Autodesk Inventor part; units mm, degrees
ref_plane "YZ Plane" through (0, 0, 0) normal (1, 0, 0) x (0, 1, 0)
ref_plane "XZ Plane" through (0, 0, 0) normal (0, 1, 0) x (-1, 0, 0)
ref_plane "XY Plane" through (0, 0, 0) normal (0, 0, 1) x (1, 0, 0)
sketch "Sketch1" plane through (0, 0, 0) normal (0, 0, 1) x (1, 0, 0)
  circle A0 centre (0, 0) radius 37.5
  dimension "d0" = 75
extrude "Extrusion1" add sketch "Sketch1" along normal blind 1
sketch "Sketch2" plane through (0, 0, 1) normal (0, 0, 1) x (1, 0, 0)
  line L0 (-10, -10) -> (10, -10)
  line L1 (10, -10) -> (10, 10)
  line L2 (10, 10) -> (-10, 10)
  line L3 (-10, 10) -> (-10, -10)
  line L4 (-10, 10) -> (10, 10)
  line L5 (10, 10) -> (10, 36.1421)
  line L6 (-10, 36.1421) -> (-10, 10)
  line L7 (10, 10) -> (36.1421, 10)
  line L8 (36.1421, -10) -> (10, -10)
  line L9 (10, -10) -> (10, 10)
  line L10 (-10, -10) -> (10, -10)
  line L11 (10, -10) -> (10, -36.1421)
  line L12 (-10, -36.1421) -> (-10, -10)
  line L13 (-10, -10) -> (-36.1421, -10)
  line L14 (-36.1421, 10) -> (-10, 10)
  line L15 (-10, 10) -> (-10, -10)
  line L16 (35.8504, 11) -> (10, 11)
  line L17 (9, 9) -> (9, -9)
  line L18 (10, -11) -> (35.8504, -11)
  line L19 (11, 10) -> (11, 35.8504)
  line L20 (-11, 35.8504) -> (-11, 10)
  line L21 (-10, 11) -> (-35.8504, 11)
  line L22 (-35.8504, -11) -> (-10, -11)
  line L23 (-9, -9) -> (-9, 9)
  line L24 (-9, -9) -> (9, -9)
  line L25 (11, -10) -> (11, -35.8504)
  line L26 (-11, -35.8504) -> (-11, -10)
  line L27 (-9, 9) -> (9, 9)
  line L28 (9, 9) -> (9, -9)
  line L29 (9, -9) -> (-9, -9)
  line L30 (10, -10) -> (9, -9) construction
  line L31 (-9, 9) -> (-10, 10) construction
  line L32 (-10, -10) -> (-9, -9) construction
  line L33 (9, 9) -> (10, 10) construction
  circle A0 centre (0, 0) radius 37.5
  line L34 (-9, -49.0456) -> (-11, -49.0456)
  point P0 (-11, -11)
  point P1 (11, -11)
  point P2 (-11, 11)
  point P3 (11, 11)
  dimension "d3" = 20
  dimension "d4" = 20
  dimension "d5" = 1
  dimension "d6" = 1
  dimension "d7" = 1
  dimension "d8" = 1
  dimension "d9" = 1
extrude "Extrusion2" add sketch "Sketch2" along normal blind 23 contours L3 L2 L1 L0 | L12 L22 L26 L13 | L8 L25 L18 L11 | L14 L20 L21 L6 | L12 A0 L26 L22 | L26 L22 A0 L13 | L5 L16 L19 L7 | L8 A0 L18 L25 | L18 L25 A0 L11 | L21 L20 A0 L6 | L14 A0 L21 L20 | L5 A0 L19 L16 | L19 L16 A0 L7
sketch "Sketch5" plane through (0, 0, 1) normal (0, 0, 1) x (1, 0, 0)
  line L0 (10, -10) -> (10, 10)
  line L1 (36.1421, -10) -> (10, -10)
  line L2 (10, 10) -> (27, 10)
  line L3 (27, 10) -> (27, -10)
  line L4 (27, -10) -> (10, -10)
  line L5 (10, -10) -> (10, 10)
  line L6 (27, 0) -> (27.5, 0)
  line L7 (27, -6) -> (28, -6)
  line L8 (28, -6) -> (28, 6)
  line L9 (28, 6) -> (27, 6)
  line L10 (27, 6) -> (27, -6)
  line L11 (27, -6) -> (28, 6) construction
  line L12 (28, -6) -> (27, 6) construction
  line L13 (-10, 10) -> (-10, -10)
  line L14 (-10, 0) -> (-27.5, 0)
  line L15 (-28, -6) -> (-27, -6)
  line L16 (-27, -6) -> (-27, 6)
  line L17 (-27, 6) -> (-28, 6)
  line L18 (-28, 6) -> (-28, -6)
  line L19 (-28, -6) -> (-27, 6) construction
  line L20 (-27, -6) -> (-28, 6) construction
  line L21 (10, -10) -> (-10, -10)
  line L22 (0, -10) -> (0, -27.5)
  line L23 (-6, -28) -> (6, -28)
  line L24 (6, -28) -> (6, -27)
  line L25 (6, -27) -> (-6, -27)
  line L26 (-6, -27) -> (-6, -28)
  line L27 (-6, -28) -> (6, -27) construction
  line L28 (6, -28) -> (-6, -27) construction
  line L29 (10, 10) -> (-10, 10)
  line L30 (0, 10) -> (0, 27.5)
  line L31 (-6, 27) -> (6, 27)
  line L32 (6, 27) -> (6, 28)
  line L33 (6, 28) -> (-6, 28)
  line L34 (-6, 28) -> (-6, 27)
  line L35 (-6, 27) -> (6, 28) construction
  line L36 (6, 27) -> (-6, 28) construction
  point P0 (0, 0)
  dimension "d21" = 17
  dimension "d22" = 0.5
  dimension "d23" = 1
  dimension "d24" = 12
  dimension "d25" = 17.5
  dimension "d26" = 1
  dimension "d27" = 12
  dimension "d28" = 17.5
  dimension "d29" = 12
  dimension "d30" = 1
  dimension "d31" = 17.5
  dimension "d32" = 12
  dimension "d33" = 1
extrude "Extrusion5" cut sketch "Sketch5" along normal blind 93 and the other way blind 11.5 contours L25 L24 L23 L26 | L16 L15 L18 L17 | L31 L34 L33 L32 | L3 L9 L8 L7
sketch "Sketch6" plane through (10, -10, 1) normal (1, 0, 0) x (0, 0, -1)
  line L0 (-7.5, 9) -> (-7.5, 11)
  line L1 (-7.5, 10) -> (0, 10)
  line L2 (0, 20) -> (0, 0)
  line L3 (0, 10) -> (-2, 10)
  line L4 (-3, 14) -> (-1, 14)
  line L5 (-1, 14) -> (-1, 6)
  line L6 (-1, 6) -> (-3, 6)
  line L7 (-3, 6) -> (-3, 14)
  line L8 (-3, 14) -> (-1, 6) construction
  line L9 (-1, 14) -> (-3, 6) construction
  point P0 (1, 10)
  dimension "d36" = 2
  dimension "d37" = 2
  dimension "d38" = 8
extrude "Extrusion6" cut sketch "Sketch6" against normal blind 23
sketch "Sketch7" plane through (-10, -10, 1) normal (0, -1, 0) x (1, 0, 0)
  line L0 (11, 7.5) -> (9, 7.5)
  line L1 (10, 7.5) -> (10, -0.0458)
  line L2 (10, -0.0458) -> (10, 1.9542)
  line L3 (6, 2.9542) -> (14, 2.9542)
  line L4 (14, 2.9542) -> (14, 0.9542)
  line L5 (14, 0.9542) -> (6, 0.9542)
  line L6 (6, 0.9542) -> (6, 2.9542)
  line L7 (6, 2.9542) -> (14, 0.9542) construction
  line L8 (14, 2.9542) -> (6, 0.9542) construction
  point P0 (10, -1)
  dimension "d41" = 2
  dimension "d42" = 8
extrude "Extrusion7" cut sketch "Sketch7" against normal blind 23
sketch "Sketch8" plane through (-10, -10, 1) normal (0, -1, 0) x (1, 0, 0)
  line L0 (6, 0.9542) -> (6, 2.9542)
  line L1 (4, 0) -> (16, 0)
  line L2 (6, 2.9542) -> (14, 2.9542)
  line L3 (14, 2.9542) -> (14, 0)
  line L4 (14, 0) -> (6, 0)
  line L5 (6, 0) -> (6, 2.9542)
  line L6 (6, 0) -> (14, 0)
  line L7 (14, 0) -> (14, 4)
  line L8 (14, 4) -> (6, 4)
  line L9 (6, 4) -> (6, 0)
  point P0 (10, -1)
  dimension "d45" = 8
  dimension "d46" = 8
  dimension "d47" = 4
extrude "Extrusion8" cut sketch "Sketch8" against normal blind 23
sketch "Sketch9" plane through (10, -10, 1) normal (1, 0, 0) x (0, 0, -1)
  line L0 (-3, 14) -> (-3, 6)
  line L1 (-3, 14) -> (0, 14)
  line L2 (0, 14) -> (0, 6)
  line L3 (0, 6) -> (-3, 6)
  line L4 (-3, 6) -> (-3, 14)
  line L5 (0, 6) -> (-4, 6)
  line L6 (-4, 6) -> (-4, 14)
  line L7 (-4, 14) -> (0, 14)
  line L8 (0, 14) -> (0, 6)
  point P0 (1, 10)
  dimension "d50" = 3
  dimension "d51" = 8
  dimension "d52" = 4
extrude "Extrusion9" cut sketch "Sketch9" against normal blind 23
sketch "Sketch10" plane through (0, 0, 24) normal (0, 0, 1) x (1, 0, 0)
  line L0 (42, 25.5) -> (-42, 25.5)
  line L1 (-42, 25.5) -> (-42, -25.5)
  line L2 (-42, -25.5) -> (42, -25.5)
  line L3 (42, -25.5) -> (42, 25.5)
  line L4 (42, 25.5) -> (-42, -25.5) construction
  line L5 (-42, 25.5) -> (42, -25.5) construction
  point P0 (0, 0)
  dimension "d55" = 84
  dimension "d56" = 51
extrude "Extrusion10" add sketch "Sketch10" along normal blind 1
sketch "Sketch11" plane through (0, 0, 25) normal (0, 0, 1) x (1, 0, 0)
  line L0 (11, -25.5) -> (42, -25.5)
  line L1 (-42, 25.5) -> (42, 25.5)
  line L2 (42, 25.5) -> (42, -25.5)
  line L3 (42, -25.5) -> (-42, -25.5)
  line L4 (-42, -25.5) -> (-42, 25.5)
  line L5 (-42, 25.5) -> (42, -25.5) construction
  line L6 (42, 25.5) -> (-42, -25.5) construction
  line L7 (43, -26.5) -> (43, 26.5)
  line L8 (43, 26.5) -> (-43, 26.5)
  line L9 (-43, 26.5) -> (-43, -26.5)
  line L10 (-43, -26.5) -> (43, -26.5)
  point P0 (0, 0)
  dimension "d59" = 1
extrude "Extrusion11" add sketch "Sketch11" along normal blind 10 and the other way blind 1
sketch "Sketch12" plane through (0, 0, 25) normal (0, 0, 1) x (1, 0, 0)
  line L0 (9, -9) -> (-9, -9)
  line L1 (-9, -9) -> (-9, 9)
  line L2 (-9, 9) -> (9, 9)
  line L3 (9, 9) -> (9, -9)
  line L4 (9, -9) -> (-9, 9) construction
  line L5 (-9, -9) -> (9, 9) construction
  point P0 (0, 0)
  dimension "d64" = 18
  dimension "d65" = 18
extrude "Extrusion12" cut sketch "Sketch12" against normal blind 10
sketch "Sketch13" plane through (0, 0, 0) normal (0, 0, -1) x (-1, 0, 0)
  line L0 (-6, 27) -> (6, 27)
  line L1 (6, 27) -> (6, 28)
  line L2 (-6, 27) -> (6, 27)
  line L3 (6, 27) -> (6, 28)
  line L4 (6, 28) -> (-6, 28)
  line L5 (-6, 28) -> (-6, 27)
  line L6 (-28, -6) -> (-28, 6)
  line L7 (-28, 6) -> (-27, 6)
  line L8 (-28, -6) -> (-27, -6)
  line L9 (-27, -6) -> (-27, 6)
  line L10 (-27, 6) -> (-28, 6)
  line L11 (-28, 6) -> (-28, -6)
  line L12 (6, -28) -> (6, -27)
  line L13 (6, -28) -> (-6, -28)
  line L14 (-6, -28) -> (-6, -27)
  line L15 (-6, -27) -> (6, -27)
  line L16 (6, -27) -> (6, -28)
  line L17 (28, 6) -> (28, -6)
  line L18 (27, 6) -> (28, 6)
  line L19 (28, -6) -> (27, -6)
  line L20 (27, -6) -> (27, 6)
  line L21 (27, 6) -> (28, 6)
  line L22 (28, 6) -> (28, -6)
  point P0 (0, 0)
extrude "Extrusion13" cut sketch "Sketch13" along normal mid plane 93
sketch "Sketch14" plane through (43, -26.5, 35) normal (1, 0, 0) x (0, 0, -1)
  line L0 (11, 16.5) -> (11, 36.5)
  line L1 (11, 26.5) -> (0, 26.5)
  line L2 (0, 0) -> (0, 53)
  line L3 (21, 34) -> (1, 34)
  line L4 (1, 34) -> (1, 19)
  line L5 (1, 19) -> (21, 19)
  line L6 (21, 19) -> (21, 34)
  line L7 (21, 34) -> (1, 19) construction
  line L8 (1, 34) -> (21, 19) construction
  line L9 (0, 19) -> (10, 19)
  line L10 (10, 19) -> (10, 34)
  line L11 (10, 34) -> (0, 34)
  line L12 (0, 34) -> (0, 19)
  point P0 (35, 26.5)
  dimension "d72" = 20
  dimension "d73" = 15
  dimension "d74" = 10
extrude "Extrusion14" cut sketch "Sketch14" against normal blind 3 contours L5 L4 L1 L10 | L1 L4 L3 L10 | L9 L2 L1 L4 | L1 L2 L11 L4
properties part number "_3DPrint"
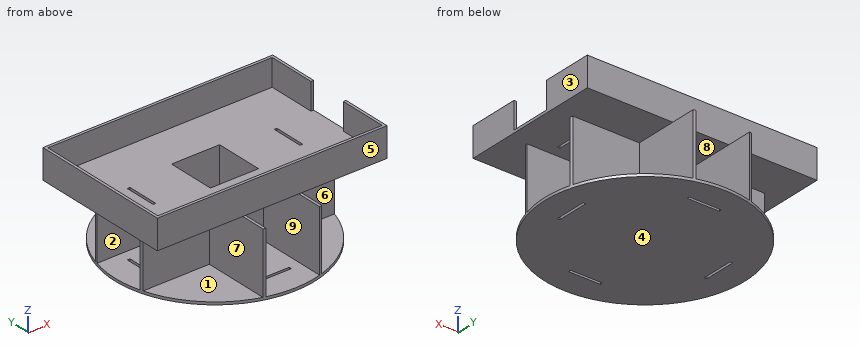
Work out the finished part from the listing and answer in its coordinate system (mm). Face numbers are marked on the shaded views. A direction names the side the tool comes from. Coordinates: 2 decimals unless noted, no trailing zeros. Write each loop counter-clockwise with the first axis right and the second up, starting at its lowest first coordinate (ties: lowest second). Pieces come first, ordered by that corner, then holes. Notation, with made-up numbers: M 85.25,2 L 125.25,2 A27 cw 125.25,18 Z; hole C 61,26 d3. An arc over 180 degrees is marked long. Write item = value, one per line.
1. The part is cut by section A-A (x = 0). Determine the outline of the cut face in (y, z), then the cut area to 3 significant figures.
Solution:
outline = M -37.5,0 L -28,0 L -28,1 L -37.5,1 Z; M -27,0 L 27,0 L 27,1 L -27,1 Z; M -26.5,24 L -10,24 L -10,5 L -9,5 L -9,25 L -25.5,25 L -25.5,35 L -26.5,35 Z; M 9,5 L 10,5 L 10,24 L 26.5,24 L 26.5,35 L 25.5,35 L 25.5,25 L 9,25 Z; M 28,0 L 37.5,0 L 37.5,1 L 28,1 Z
area = 166 mm2
2. Determine the mould class of the marked faces 1, 2, 3 and 4 for opening direction Z: released by +Z, released by -Z, zero draft, split by the parting line, or undercut.
Solution:
face_1 = undercut
face_2 = undercut
face_3 = zero draft
face_4 = released by -Z
3. Straight lines are drawn through the part: line 1 (X direction, y = -8.5, z = 21.5); line 2 (Y direction, x = -34, z = 26); line 3 (Z direction, x = 0, y = -17.5). For each, find the intervals that lie inside material, in ascending order. Write a range as from..to.
Solution:
line_1 = -10..-9, 9..10
line_2 = -26.5..-25.5, 25.5..26.5
line_3 = 0..1, 24..25
4. The part is cut by section D-D (x = -12.5). Determine the outline of the cut face in (y, z), then the cut area to 3 significant figures.
Solution:
outline = M -35.36,0 L 35.36,0 L 35.36,1 L 11,1 L 11,24 L 26.5,24 L 26.5,35 L 25.5,35 L 25.5,25 L -25.5,25 L -25.5,35 L -26.5,35 L -26.5,24 L -11,24 L -11,1 L -35.36,1 Z; hole M -10,1 L 10,1 L 10,24 L -10,24 Z
area = 190 mm2
5. For the marked faces 5, 6, 7, 8 and 9, determine the directions among +Z, -Z, +X, -X, +Y, -Y from which every point of the face is accessible in a straight line to the end or side of a thin tool.
Solution:
face_5 = +Z, +X, -X, -Y
face_6 = +X, -Y
face_7 = -X, -Y
face_8 = +Y
face_9 = -Y
6. Flat-ended cylindrical pins translate along their axes: pin 1 (6 mm diameter, centred on x = 12.5, z = 31, fed in from -Y); pin 2 (10 mm diameter, centred on x = -3, z = 21, fed in from +Y); pin 3 (10 mm diameter, centred on x = -33, z = 17, fed in from +Y). Find the tip coordinate at first contact, or state that the pin passes through.
Solution:
pin_1 = -26.5
pin_2 = 26.5
pin_3 = 11
